Design review of the part shown in the three views and the two pictorial views. Dimensions are in mm from the part's minimum x, y and z. Coordinates: 2 decimals unless noted, no trailing zeros. Order: outer loops, then holes, each group sorted by start corner. A loop starts at its lowest first (then second) coordinate and runs counter-clockwise, first axis right, second up. Notation, with made-up numbers: (23, -17.5) -> (35, -17.5) arc R21 cw to (35, -6.5) -> close; hole circle Ø10 at (41.5, 75.5). An arc over 180 degrees is marked (long way). Write item = value, one per line. Start each with the question number.
1) Wall thickness on probe 1 along Y at (x, z) = (75, 1.2); probe 2 along Y at (x, z) = (25, 0.75); probe 3 along X at (y, z) = (90, 1.65): over which ranges is each line inside the solid? List them lowest first. Write a range as [from, to].
2) Consider section B-B on x = 75. Give the boundary of the cut face in (y, z), and give its area (3 significant figures).
3) Consider section C-C on y = 60. Give the boundary of the cut face in (x, z).
4) Consider section A-A on z = 1.35. State how many separate pieces and enclosed holes the cut face has, and give its area (3 significant figures).
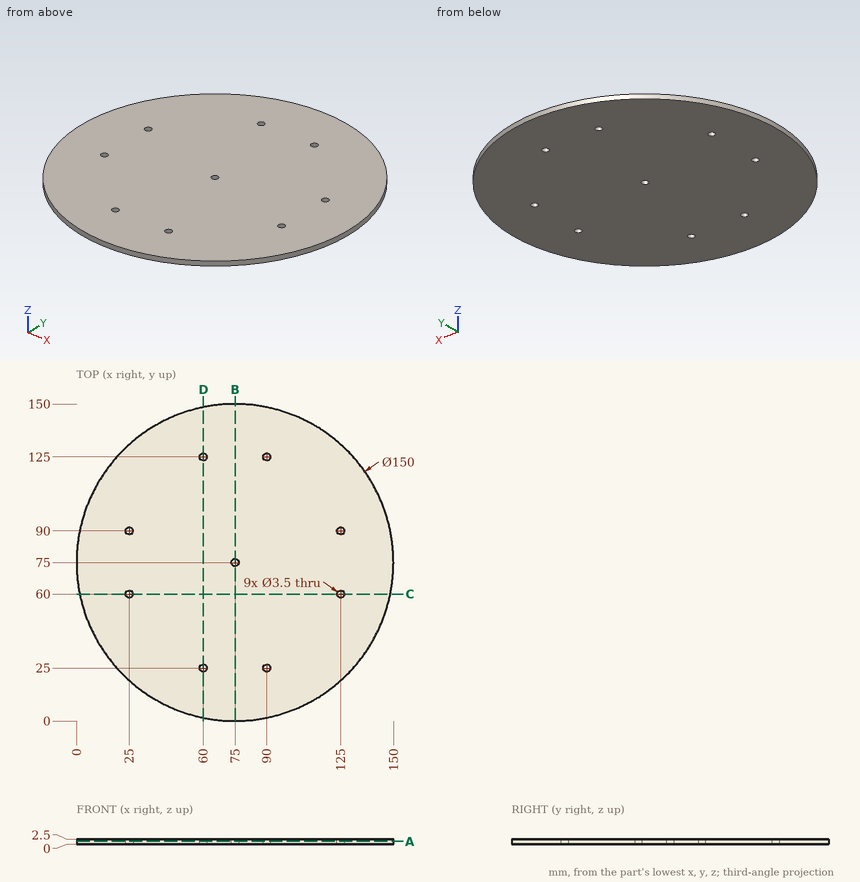
Answer sheet:
q1.probe_1 = [0, 73.25], [76.75, 150]
q1.probe_2 = [19.1, 58.25], [61.75, 88.25], [91.75, 130.9]
q1.probe_3 = [1.52, 23.25], [26.75, 123.25], [126.75, 148.48]
q2.outline = (0, 0) -> (73.25, 0) -> (73.25, 2.5) -> (0, 2.5) -> close; (76.75, 0) -> (150, 0) -> (150, 2.5) -> (76.75, 2.5) -> close
q2.area = 366 mm2
q3.outline = (1.52, 0) -> (23.25, 0) -> (23.25, 2.5) -> (1.52, 2.5) -> close; (26.75, 0) -> (123.25, 0) -> (123.25, 2.5) -> (26.75, 2.5) -> close; (126.75, 0) -> (148.48, 0) -> (148.48, 2.5) -> (126.75, 2.5) -> close
q4.separate_pieces = 1
q4.enclosed_holes = 9
q4.area = 17,600 mm2
